Read the model definition and answer for the solid it produces. Units are mm, in the model's axes. Face numbers are marked on the shaded views. A direction names the side the tool comes from. Give positions to 0.01 mm unless a question says otherwise; leave off trailing zeros. Loops run counter-clockwise (first coordinate to the right, second up) from the corner with the lowest first, then second, coordinate; pieces in that order, holes last. Notation, with made-up numbers: (30, 51) - (48, 51) arc R29 cw to (48, 75) - close; hole circle Ø5 at (-32.5, 67). An arc over 180 degrees is marked (long way). Write item = value, one per line.
Solid Edge part; units mm, degrees
sketch "Sketch1" plane through (0, 0, 0) normal (0, 0, 1) x (1, 0, 0)
  line L0 (-10.9265, -1.0891) -> (14.4735, -1.0891)
  line L1 (14.4735, -1.0891) -> (14.4735, 5.2609)
  line L2 (14.4735, 5.2609) -> (-10.9265, 5.2609)
  line L3 (-10.9265, 5.2609) -> (-10.9265, -1.0891)
extrude "Protrusion1" add sketch "Sketch1" along normal blind 2.5
sketch "Sketch2" plane through (1.7735, 2.0859, 2.5) normal (0, 0, 1) x (0, 1, 0)
  line L0 (-3.175, -1.8) -> (-3.175, -6.5)
  line L1 (-3.175, -6.5) -> (3.175, -6.5)
  line L2 (3.175, -6.5) -> (3.175, -1.8)
  line L3 (-3.175, -1.8) -> (3.175, -1.8)
  line L4 (3.175, 1.8) -> (3.175, 6.5)
  line L5 (-3.175, 6.5) -> (3.175, 6.5)
  line L6 (-3.175, 6.5) -> (-3.175, 1.8)
  line L7 (-3.175, 1.8) -> (3.175, 1.8)
extrude "ExtrudedProtrusion_2" add sketch "Sketch2" along normal blind 9.2
fillet "Round_1" radius 0.1 2 edges at (-4.7265, 2.0859, 2.5) (8.2735, 2.0859, 2.5)
fillet "Round_2" radius 1.8 2 edges at (-0.0265, 2.0859, 2.5) (3.5735, 2.0859, 2.5)
sketch "Sketch3" plane through (1.7735, 2.0859, 0) normal (0, 0, -1) x (1, 0, 0)
  line L0 (-3.935, 2.02) -> (-3.935, 0.52)
  line L1 (-3.935, 0.52) -> (-3.685, 0.52)
  line L2 (-3.685, 0.52) -> (-3.685, 2.02)
  line L3 (-3.685, 2.02) -> (-3.935, 2.02)
  line L4 (-3.935, -0.52) -> (-3.685, -0.52)
  line L5 (-3.685, -0.52) -> (-3.685, -2.02)
  line L6 (-3.685, -2.02) -> (-3.935, -2.02)
  line L7 (-3.935, -2.02) -> (-3.935, -0.52)
  line L8 (3.935, -2.02) -> (3.935, -0.52)
  line L9 (3.935, -0.52) -> (3.685, -0.52)
  line L10 (3.685, -0.52) -> (3.685, -2.02)
  line L11 (3.685, -2.02) -> (3.935, -2.02)
  line L12 (3.935, 0.52) -> (3.685, 0.52)
  line L13 (3.685, 0.52) -> (3.685, 2.02)
  line L14 (3.685, 2.02) -> (3.935, 2.02)
  line L15 (3.935, 2.02) -> (3.935, 0.52)
extrude "ExtrudedProtrusion_3" add sketch "Sketch3" along normal blind 6.5
sketch "Sketch4" plane through (-4.7265, 2.0859, 8.55) normal (-1, 0, 0) x (0, -1, 0)
  circle A0 centre (0, 0.05) radius 1.25
extrude "Cutout1" cut sketch "Sketch4" against normal through all
sketch "Sketch5" plane through (1.7735, 2.0859, 0) normal (0, 0, -1) x (1, 0, 0)
  circle A0 centre (-9.5, 0) radius 1.6
  circle A1 centre (9.5, 0) radius 1.6
extrude "Cutout2" cut sketch "Sketch5" against normal through all
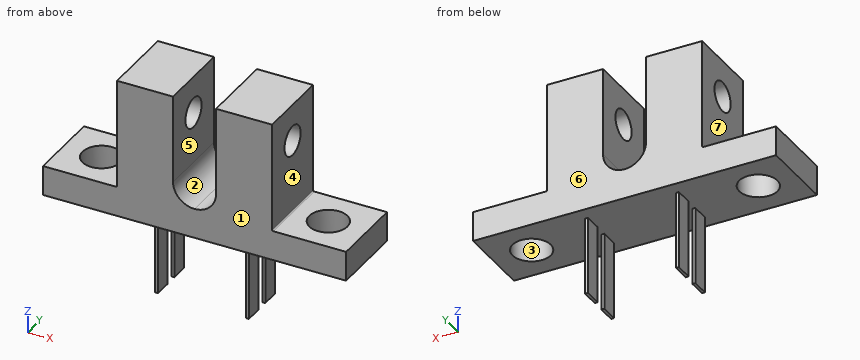
1) A cutting plane is placed at D-D on x = -4.25. Determine the outline of the cut face in (y, z), then the cut area to 3 significant figures.
Output:
outline = (-1.09, 0) - (5.26, 0) - (5.26, 11.7) - (-1.09, 11.7) - close; hole circle Ø2.5 at (2.09, 8.6)
area = 69.4 mm²
2) A cutting plane is placed at A-A on z = -2.75. Determine the outline of the cut face in (x, y).
Output:
outline = (-2.16, 0.07) - (-1.91, 0.07) - (-1.91, 1.57) - (-2.16, 1.57) - close; (-2.16, 2.61) - (-1.91, 2.61) - (-1.91, 4.11) - (-2.16, 4.11) - close; (5.46, 0.07) - (5.71, 0.07) - (5.71, 1.57) - (5.46, 1.57) - close; (5.46, 2.61) - (5.71, 2.61) - (5.71, 4.11) - (5.46, 4.11) - close
3) Each of these flat-tipped pins is pushed along its axis until it touches: P1, Ø0.8, axis at y = 3, z = -2.5, coming from the -X side; P2, Ø4, axis at x = 9.5, z = -4, coming from the +Y side; P3, Ø1.9, axis at y = 2, z = 5.5, coming from the +X side; P4, Ø0.8, axis at y = 3.5, z = -4.5, coming from the +X side. Where does it stop, or does it pass through?
Output:
P1 = -2.16
P2 = through
P3 = 8.27
P4 = 5.71
4) A tool of negligible diameter and unlimited length cuts with its end or side. For the marked faces 4, 5, 6 and 7, from which of +Z, -Z, +X, -X, +Y, -Y can it reach the whole face along a straight path? Write none if from no direction.
Output:
face_4 = +Z, +X, +Y, -Y
face_5 = +Z, +Y, -Y
face_6 = +Z, -Z, +X, -X, +Y
face_7 = +Z, -X, +Y, -Y
5) A cutting plane is placed at B-B on x = 11.5. Determine the outline of the cut face in (y, z).
Output:
outline = (-1.09, 0) - (0.5, 0) - (0.5, 2.5) - (-1.09, 2.5) - close; (3.67, 0) - (5.26, 0) - (5.26, 2.5) - (3.67, 2.5) - close
6) Find the intervals of material crossed by probe 1 along X at (y, z) = (5, 5); probe 2 along Z at (x, y) = (-9.5, 3.75); probe 3 along Z at (x, y) = (6.5, 4.75), in increasing order.
Output:
probe_1 = -4.73 to -0.03, 3.57 to 8.27
probe_2 = 0 to 2.5
probe_3 = 0 to 11.7
7) The mould has two halves that part along Y. Classify the marked faces 1, 2 and 3: pulls with the +Y half, pulls with the -Y half, needs draft (parallel to the pull), parting line crosses it, or undercut.
Output:
face_1 = pulls with the -Y half
face_2 = needs draft
face_3 = undercut
